Verification items for this drawing (mm, ordinates from the low corner). A direction names the side the tool comes from. Round coordinates to 2 decimals unless told otherwise and drop trailing zeros. One line per question, with ' | ' between items. Start each with the question number.
Q1. Tool access check on the marked faces 1 and 2. Record the directions out of +Z, -Z, +X, -X, +Y, -Y that give a thin tool (end or side, any length) a straight path to the whole face; none if there is none.
Q2. Gauge pin test, flat ends, axial feed: pin 1 (4 mm diameter, centred on x = 17, z = 21.5, fed in from +Y); pin 2 (8 mm diameter, centred on x = 6, z = 19.5, fed in from +Y); pin 3 (2 mm diameter, centred on x = 17, z = 20.5, fed in from -Y). Record the tip position at first contact, or that the pin passes through.
Q3. Thickness scan on line 1 along X through (y, z) = (46.5, 20.5); line 2 along Y through (x, z) = (9.25, 15.5); line 3 along Y through (x, z) = (5.5, 9.5). Record the ranges inside material, lowest first. Write a range as from..to.
Q4. Release check for a two-part mould opening along Y. For the marked faces 3, 4 and 5 record: released by +Y, released by -Y, zero draft, split by the parting line, or undercut.
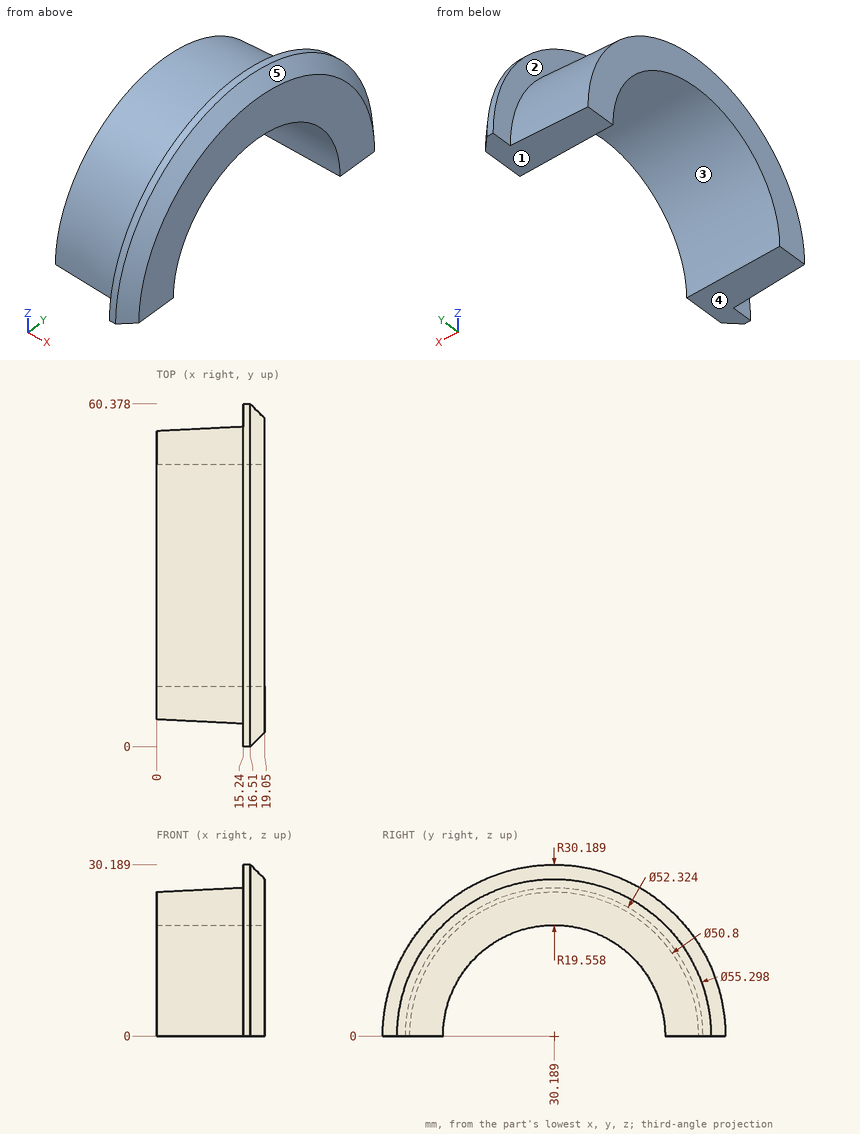
Determined:
1) face 1: -Z, +X, -X, +Y, -Y | face 2: +Z, -X
2) pin 1: stops at y = 53.18 | pin 2: stops at y = 50.7 | pin 3: stops at y = 7.25
3) line 1: x = 15.24..19.05 | line 2: y = 9.49..18.26, 42.12..50.89 | line 3: y = 6.34..13.09, 47.28..54.04
4) face 3: undercut | face 4: zero draft | face 5: split by the parting line
